Verification items for the finished model (mm, model axes). Face numbers are marked on the shaded views. A direction names the side the tool comes from. Give positions to 0.01 mm unless a question says otherwise; leave off trailing zeros. Order: outer loops, then holes, each group sorted by start corner. A loop starts at its lowest first (then second) coordinate and runs counter-clockwise, first axis right, second up. Notation, with made-up numbers: (34, 14.25) -> (76, 14.25) arc R20 cw to (76, 52.25) -> close; hole circle Ø8 at (60, 50). An arc over 180 degrees is marked (long way). Write each question's results on one line, items separated by ' | '. Start each with the question number.
1. Cross-section at C-C, the plane x = 6.5. Enter the section's corners in (y, z).
2. Cross-section at B-B, the plane y = 18. Enter the section's corners in (x, z), then the cut area to 3 significant figures.
3. Mould release check, pull along X, two halves, no side actions. Record for the marked faces 1, 2, 3 and 4: +X half, -X half, draft (parallel to the pull), parting line (faces both ways), or undercut.
4. Cross-section at D-D, the plane z = 14. Enter the section's corners in (x, y).
5. Set-up check for the marked faces 5 and 6: record each of +Z, -Z, +X, -X, +Y, -Y from which the full face is reachable in a straight line by a thin tool's end or side.
6. Cross-section at A-A, the plane x = 38.5. Enter the section's corners in (y, z), then the cut area to 3 significant figures.
7. Depth check by flat-ended pin: pin 1 Ø10 at (x, y) = (25, -13) entering from +Z; pin 2 Ø1.3 at (x, y) = (49.5, 4.5) entering from +Z. Enter the tip coordinate at first touch or a pass-through.
8. Material ranges on L1, parallel to X at y = -12.5, z = 11.5; L2, parallel to Y at x = 10, z = 4; L3, parallel to Z at x = 29, y = -27, recorded low to high. Write a range as from..to.
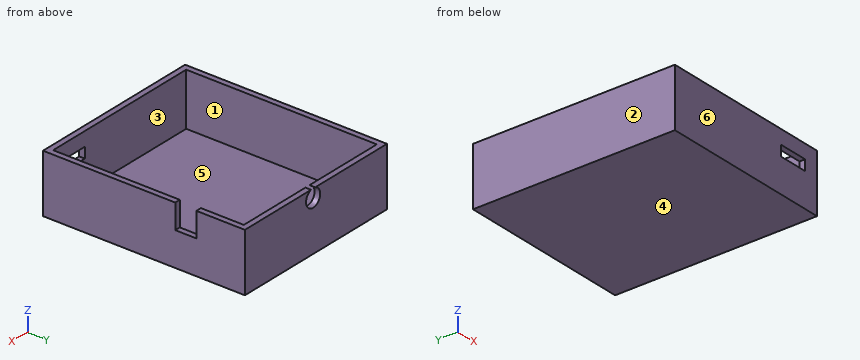
from build123d import *

# Parameters (mm, degrees)
SKETCH1_W           = 50.2
SKETCH1_H           = 57.4
BOSS_EXTRUDE1_DEPTH = 16.6
SHELL1_T            = -1.6
SKETCH2_W           = 8.6
SKETCH2_H           = 3
CUT_EXTRUDE1_DEPTH  = 16.6
SKETCH3_W           = 9.2
SKETCH3_H           = 6
CUT_EXTRUDE2_DEPTH  = 16.6
SKETCH4_R           = 2.5
CUT_EXTRUDE3_DEPTH  = 16.6


with BuildPart() as part:
    # Sketch1 → Boss-Extrude1 (new body)
    with BuildSketch(Plane.XY):
        with Locations((25.1, -5.901746725)):
            Rectangle(SKETCH1_W, SKETCH1_H)
    extrude(amount=BOSS_EXTRUDE1_DEPTH)

    # Shell1
    shell1_openings = [part.faces().sort_by_distance(p)[0] for p in [
        (25.1, -5.901746725, 16.6),
    ]]
    offset(amount=SHELL1_T, openings=shell1_openings, kind=Kind.INTERSECTION)

    # Sketch2 → Cut-Extrude1 (cut)
    with BuildSketch(Plane.XZ.offset(34.601746725)):
        with Locations((41.7, 11.1)):
            Rectangle(SKETCH2_W, SKETCH2_H)
    extrude(amount=-CUT_EXTRUDE1_DEPTH, mode=Mode.SUBTRACT)

    # Sketch3 → Cut-Extrude2 (cut)
    with BuildSketch(Plane(origin=(50.2, 0, 0), x_dir=(0, 0, -1), z_dir=(1, 0, 0))):
        with Locations((-14.2, 5.998253275)):
            Rectangle(SKETCH3_W, SKETCH3_H)
    extrude(amount=-CUT_EXTRUDE2_DEPTH, mode=Mode.SUBTRACT)

    # Sketch4 → Cut-Extrude3 (cut)
    with BuildSketch(Plane(origin=(0, 22.798253275, 0), x_dir=(1, 0, 0), z_dir=(0, 1, 0))):
        with Locations((26.1, -14.206462085)):
            Circle(SKETCH4_R)
    extrude(amount=-CUT_EXTRUDE3_DEPTH, mode=Mode.SUBTRACT)


solid = part.part
Results below:
1) outline: (-34.6, 0) -> (22.8, 0) -> (22.8, 16.6) -> (21.2, 16.6) -> (21.2, 1.6) -> (-33, 1.6) -> (-33, 16.6) -> (-34.6, 16.6) -> close
2) outline: (0, 0) -> (50.2, 0) -> (50.2, 16.6) -> (48.6, 16.6) -> (48.6, 1.6) -> (1.6, 1.6) -> (1.6, 16.6) -> (0, 16.6) -> close | area: 128 mm²
3) face 1: undercut | face 2: -X half | face 3: undercut | face 4: draft
4) outline: (0, -34.6) -> (50.2, -34.6) -> (50.2, 3) -> (48.6, 3) -> (48.6, -33) -> (1.6, -33) -> (1.6, 21.2) -> (23.61, 21.2) -> (23.61, 22.8) -> (0, 22.8) -> close; (28.59, 21.2) -> (48.6, 21.2) -> (48.6, 9) -> (50.2, 9) -> (50.2, 22.8) -> (28.59, 22.8) -> close
5) face 5: +Z | face 6: +Z, -Z, +X, -X, -Y
6) outline: (-34.6, 0) -> (22.8, 0) -> (22.8, 16.6) -> (21.2, 16.6) -> (21.2, 1.6) -> (-33, 1.6) -> (-33, 9.6) -> (-34.6, 9.6) -> close; (-34.6, 12.6) -> (-33, 12.6) -> (-33, 16.6) -> (-34.6, 16.6) -> close | area: 135 mm²
7) pin 1: stops at z = 1.6 | pin 2: stops at z = 9.6
8) L1: x = 0..1.6, 48.6..50.2 | L2: y = -34.6..-33, 21.2..22.8 | L3: z = 0..1.6
